Can you work these out from the model? Positions are in its coordinate system, mm. A direction names the side the tool comes from. Round coordinates to 2 decimals unless told otherwise and drop trailing zeros. Write each loop counter-clockwise with the first axis right and the second up, starting at its lowest first coordinate (ties: lowest second). Pieces come first, ordered by that corner, then holes. Notation, with made-up numbers: (64.25, 82) -> (87.25, 82) arc R21 cw to (87.25, 92) -> close; hole circle Ø3 at (61.25, 34). An arc over 180 degrees is marked (long way). Write item = value, one per line. Start each with the question number.
1) I'm going to push flat-ended pins straight in: pin 1 (3.5 mm diameter, centred on x = 32.58, z = 35.77, fed in from -Y); pin 2 (5 mm diameter, centred on x = 23.5, z = 56.5, fed in from -Y) (3 decimals). Where does each tip first touch, or does it pass through?
2) For faces 4 (the face through (1, 3.175, -1)), 5 (the face through (-1, 9.525, -1)), 6 (the face through (-88.9, 6, 1)), which set-ups out of +Z, -Z, +X, -X, +Y, -Y let a thin tool reach every point of the face, with its end or its side?
3) Imagine slicing it at B-B, the plane x = 46. Please give me the cut outline in (y, z) (3 decimals).
4) Imagine slicing it at A-A, the plane z = 21.5. Please give me the cut outline in (x, y) (3 decimals), then the cut area to 3 significant figures.
5) If I drill on line 1 (Z direction, x = 34.5, y = 7.5); line 2 (Z direction, x = -34, y = 4); line 3 (Y direction, x = -42, z = 27) (3 decimals), over which ranges is the centre line in solid material (lowest first)?
6) Thinking about a two-plate mould opening in Z: for faces 1 (the face through (-37.673, 6.394, 35.166)), 2 (the face through (-1, 6, -88.9)), 3 (the face through (-1, 6, 88.9)), which applies, +Z half, -Z half, draft (parallel to the pull), parting line (faces both ways), or undercut?
from build123d import *

# Parameters (mm, degrees)
SKETCH10_W          = 177.8
SKETCH10_H          = 177.8
BOSS_EXTRUDE4_DEPTH = 12.7
SKETCH12_W          = 127
SKETCH12_H          = 127
BOSS_EXTRUDE5_DEPTH = 3.175
SKETCH13_W          = 127
SKETCH13_H          = 127
CUT_EXTRUDE1_DEPTH  = 3.175
SKETCH14_W          = 127
SKETCH14_H          = 127
CUT_EXTRUDE2_DEPTH  = 3.175
FILLET4_R           = 2.54
SKETCH16_R          = 2.794
CUT_EXTRUDE3_DEPTH  = 25.4


with BuildPart() as part:
    # Sketch10 → Boss-Extrude4 (new body)
    with BuildSketch(Plane(origin=(0, 0, 0), x_dir=(1, 0, 0), z_dir=(0, 1, 0))):
        Rectangle(SKETCH10_W, SKETCH10_H)
    extrude(amount=BOSS_EXTRUDE4_DEPTH)

    # Sketch12 → Boss-Extrude5 (add)
    with BuildSketch(Plane(origin=(0, 12.7, 0), x_dir=(1, 0, 0), z_dir=(0, 1, 0))):
        Rectangle(SKETCH12_W, SKETCH12_H)
    extrude(amount=-BOSS_EXTRUDE5_DEPTH)

    # Sketch13 → Cut-Extrude1 (cut)
    with BuildSketch(Plane(origin=(0, 12.7, 0), x_dir=(1, 0, 0), z_dir=(0, 1, 0))):
        Rectangle(SKETCH13_W, SKETCH13_H)
    extrude(amount=-CUT_EXTRUDE1_DEPTH, mode=Mode.SUBTRACT)

    # Sketch14 → Cut-Extrude2 (cut)
    with BuildSketch(Plane(origin=(0, 0, 0), x_dir=(-1, 0, 0), z_dir=(0, -1, 0))):
        Rectangle(SKETCH14_W, SKETCH14_H)
    extrude(amount=-CUT_EXTRUDE2_DEPTH, mode=Mode.SUBTRACT)

    # Fillet4
    fillet4_edges = [part.edges().sort_by_distance(p)[0] for p in [
        (-63.5, 9.525, 0),
        (0, 9.525, -63.5),
        (63.5, 9.525, 0),
        (0, 9.525, 63.5),
        (63.5, 3.175, 0),
        (0, 3.175, -63.5),
        (-63.5, 3.175, 0),
        (0, 3.175, 63.5),
    ]]
    fillet(fillet4_edges, radius=FILLET4_R)

    # Sketch16 → Cut-Extrude3 (cut)
    with BuildSketch(Plane(origin=(0, 9.525, 0), x_dir=(1, 0, 0), z_dir=(0, 1, 0))):
        with Locations(Location((-34.945581996, 36.952591773, 0), (0, 0, 270))):
            Circle(SKETCH16_R)
        with Locations(Location((32.584394023, 36.952591773, 0), (0, 0, 270))):
            Circle(SKETCH16_R)
        with Locations(Location((-34.945581996, -35.771997786, 0), (0, 0, 270))):
            Circle(SKETCH16_R)
        with Locations(Location((32.584394023, -35.771997786, 0), (0, 0, 270))):
            Circle(SKETCH16_R)
    extrude(amount=-CUT_EXTRUDE3_DEPTH, mode=Mode.SUBTRACT)


solid = part.part
Reported:
q1.pin_1 = through
q1.pin_2 = 3.175
q2.face_4 = -Y
q2.face_5 = +Y
q2.face_6 = +Z, -Z, -X, +Y, -Y
q3.outline = (0, -88.9) -> (12.7, -88.9) -> (12.7, -63.5) -> (12.065, -63.5) arc R2.54 cw to (9.525, -60.96) -> (9.525, 60.96) arc R2.54 cw to (12.065, 63.5) -> (12.7, 63.5) -> (12.7, 88.9) -> (0, 88.9) -> (0, 63.5) -> (0.635, 63.5) arc R2.54 cw to (3.175, 60.96) -> (3.175, -60.96) arc R2.54 cw to (0.635, -63.5) -> (0, -63.5) -> close
q4.outline = (-88.9, 0) -> (-63.5, 0) -> (-63.5, 0.635) arc R2.54 cw to (-60.96, 3.175) -> (60.96, 3.175) arc R2.54 cw to (63.5, 0.635) -> (63.5, 0) -> (88.9, 0) -> (88.9, 12.7) -> (63.5, 12.7) -> (63.5, 12.065) arc R2.54 cw to (60.96, 9.525) -> (-60.96, 9.525) arc R2.54 cw to (-63.5, 12.065) -> (-63.5, 12.7) -> (-88.9, 12.7) -> close
q4.area = 1,460 mm²
q5.line_1 = -88.9 to -38.99, -34.92 to 33.74, 37.81 to 88.9
q5.line_2 = -88.9 to -39.58, -34.32 to 33.14, 38.4 to 88.9
q5.line_3 = 3.175 to 9.525
q6.face_1 = undercut
q6.face_2 = -Z half
q6.face_3 = +Z half
